Here's how the part is built. I have some questions about the finished solid (model axes, mm). Face numbers are marked on the shaded views. Give positions to 0.01 mm unless a question says otherwise; leave off trailing zeros. Write each loop counter-clockwise with the first axis right and the second up, starting at its lowest first coordinate (ties: lowest second). Pieces come first, ordered by that corner, then holes. Notation, with made-up numbers: (32, 40.5) - (74, 40.5) arc R6 cw to (74, 50.5) - close; hole circle Ø11 at (22, 87.5). An arc over 180 degrees is marked (long way). One line per item, written item: value. Start each with the question number.
1) I'm going to push flat-ended pins straight in: P1, Ø12, axis at x = 405.5, z = 309.5, coming from the +Y side; P2, Ø6, axis at x = 604.5, y = 30, coming from the +Z side; P3, Ø12, axis at x = -440.5, z = 47.5, coming from the -Y side; P4, Ø1.5, axis at x = -524.5, y = 75, coming from the +Z side. Where does each tip first touch, or does it pass through?
2) Imagine slicing it at A-A on z = 0. Write out the boundary of the cut face in (x, y).
3) We'd pull the mould along Z, two halves only. Please class the marked faces 1 and 2: +Z half, -Z half, draft (parallel to the pull), parting line (faces both ways), or undercut.
4) Imagine slicing it at D-D on x = -624. Write out the boundary of the cut face in (y, z).
5) Please list where these lines run through material, in increasing order: L1, parallel to X at y = 92.5, z = 550; L2, parallel to X at y = 53, z = 0; L3, parallel to X at y = 113, z = -459.5. Write a range as [from, to].
6) Imagine slicing it at B-B on y = 39.5. Write out the boundary of the cut face in (x, z).
7) Imagine slicing it at C-C on x = 82. Write out the boundary of the cut face in (y, z), plus the area to 3 significant figures.
from build123d import *

# Parameters (mm, degrees)
IZIM1_R                     = 400
Y_KSEKLIK_EKSTR_ZYON1_DEPTH = 70
IZIM2_R                     = 135
IZIM2_R_2                   = 100
Y_KSEKLIK_EKSTR_ZYON2_DEPTH = 100


with BuildPart() as part:
    # Çizim1 → Yükseklik-Ekstrüzyon1 (new body)
    with BuildSketch(Plane(origin=(0, 0, 0), x_dir=(1, 0, 0), z_dir=(0, 1, 0))):
        with BuildLine():
            Line((800, 400), (800, -400))
            ThreePointArc((800, -400), (682.842712475, -682.842712475), (400, -800))
            Line((400, -800), (-400, -800))
            ThreePointArc((-400, -800), (-682.842712475, -682.842712475), (-800, -400))
            Line((-800, -400), (-800, 400))
            ThreePointArc((-800, 400), (-682.842712475, 682.842712475), (-400, 800))
            Line((-400, 800), (400, 800))
            ThreePointArc((400, 800), (682.842712475, 682.842712475), (800, 400))
        make_face()
        with Locations(Location((0, 0, 0), (0, 0, 270))):
            Circle(IZIM1_R, mode=Mode.SUBTRACT)
    extrude(amount=Y_KSEKLIK_EKSTR_ZYON1_DEPTH)

    # Çizim2 → Yükseklik-Ekstrüzyon2 (add)
    # profile 1 of 4: a face of its own
    with BuildSketch(Plane(origin=(0, 70, 0), x_dir=(1, 0, 0), z_dir=(0, 1, 0))):
        with Locations(Location((-550, 550, 0), (0, 0, 270))):
            Circle(IZIM2_R)
        with Locations(Location((-550, 550, 0), (0, 0, 270))):
            Circle(IZIM2_R_2, mode=Mode.SUBTRACT)
    # profile 2 of 4: a face of its own
    with BuildSketch(Plane(origin=(0, 70, 0), x_dir=(1, 0, 0), z_dir=(0, 1, 0))):
        with Locations(Location((550, 550, 0), (0, 0, 270))):
            Circle(IZIM2_R)
        with Locations(Location((550, 550, 0), (0, 0, 270))):
            Circle(IZIM2_R_2, mode=Mode.SUBTRACT)
    # profile 3 of 4: a face of its own
    with BuildSketch(Plane(origin=(0, 70, 0), x_dir=(1, 0, 0), z_dir=(0, 1, 0))):
        with Locations(Location((-550, -550, 0), (0, 0, 270))):
            Circle(IZIM2_R)
        with Locations(Location((-550, -550, 0), (0, 0, 270))):
            Circle(IZIM2_R_2, mode=Mode.SUBTRACT)
    # profile 4 of 4: a face of its own
    with BuildSketch(Plane(origin=(0, 70, 0), x_dir=(1, 0, 0), z_dir=(0, 1, 0))):
        with Locations(Location((550, -550, 0), (0, 0, 270))):
            Circle(IZIM2_R)
        with Locations(Location((550, -550, 0), (0, 0, 270))):
            Circle(IZIM2_R_2, mode=Mode.SUBTRACT)
    extrude(amount=Y_KSEKLIK_EKSTR_ZYON2_DEPTH)


solid = part.part
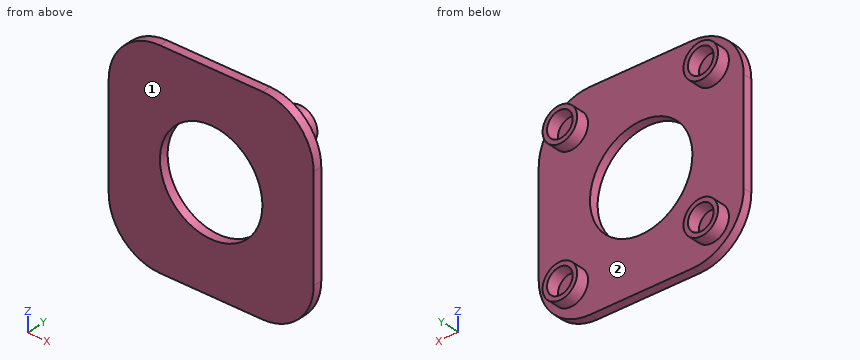
Numbers:
1. P1: y = 70
1. P2: z = 745.54
1. P3: y = 0
1. P4: z = 682.71
2. outline: (-800, 0) - (-400, 0) - (-400, 70) - (-800, 70) - close; (400, 0) - (800, 0) - (800, 70) - (400, 70) - close
3. face 1: draft
3. face 2: undercut
4. outline: (0, -731.4) - (70, -731.4) - (70, -662.91) - (170, -662.91) - (170, -617.26) - (70, -617.26) - (70, -482.74) - (170, -482.74) - (170, -437.09) - (70, -437.09) - (70, 437.09) - (170, 437.09) - (170, 482.74) - (70, 482.74) - (70, 617.26) - (170, 617.26) - (170, 662.91) - (70, 662.91) - (70, 731.4) - (0, 731.4) - close
5. L1: [-685, -650], [-450, -415], [415, 450], [650, 685]
5. L2: [-800, -400], [400, 800]
5. L3: [-650.17, -592.54], [-507.46, -449.83], [449.83, 507.46], [592.54, 650.17]
6. outline: (-800, -400) arc R400 ccw to (-400, -800) - (400, -800) arc R400 ccw to (800, -400) - (800, 400) arc R400 ccw to (400, 800) - (-400, 800) arc R400 ccw to (-800, 400) - close; hole circle Ø800 at (0, 0)
7. outline: (0, -800) - (70, -800) - (70, -391.5) - (0, -391.5) - close; (0, 391.5) - (70, 391.5) - (70, 800) - (0, 800) - close
7. area: 57,200 mm^2
